Autodesk Inventor part; units mm, degrees
ref_plane "YZ Plane" through (0, 0, 0) normal (1, 0, 0) x (0, 1, 0)
ref_plane "XZ Plane" through (0, 0, 0) normal (0, 1, 0) x (-1, 0, 0)
ref_plane "XY Plane" through (0, 0, 0) normal (0, 0, 1) x (1, 0, 0)
sketch "Sketch1" plane through (0, 0, 0) normal (0, 0, 1) x (1, 0, 0)
  line L0 (-7.5, 7.5) -> (7.5, 7.5)
  line L1 (7.5, 7.5) -> (7.5, -7.5)
  line L2 (7.5, -7.5) -> (-7.5, -7.5)
  line L3 (-7.5, -7.5) -> (-7.5, 7.5)
  line L4 (-7.5, 7.5) -> (7.5, -7.5) construction
  line L5 (7.5, 7.5) -> (-7.5, -7.5) construction
  point P0 (0, 0)
  dimension "d0" = 15
  dimension "d1" = 15
extrude "Extrusion1" add sketch "Sketch1" along normal blind 2
sketch "Sketch2" plane through (0, 0, 2) normal (0, 0, 1) x (1, 0, 0)
  line L0 (-7.5, -7.5) -> (7.5, -7.5)
  line L1 (1.5, 7.5) -> (1.5, -7.5) construction
  line L2 (-1.5, -7.5) -> (-1.5, 7.5) construction
  line L3 (1.5, 7.5) -> (2, 7.5) construction
  line L4 (2, 7.5) -> (2, -7.5)
  line L5 (2, -7.5) -> (1.5, -7.5)
  line L6 (1.5, -7.5) -> (1.5, 7.5)
  line L7 (7.5, -7.5) -> (-7.5, -7.5)
  line L8 (-1.5, 7.5) -> (-2, 7.5)
  line L9 (-2, 7.5) -> (-2, -7.5)
  line L10 (-2, -7.5) -> (-1.5, -7.5)
  line L11 (-1.5, -7.5) -> (-1.5, 7.5)
  line L12 (7.5, 7.5) -> (-7.5, 7.5)
  line L13 (2, -7.5) -> (3, -7.5)
  line L14 (3, -7.5) -> (3, 7.5)
  line L15 (3, 7.5) -> (2, 7.5)
  line L16 (-2, 7.5) -> (-3, 7.5)
  line L17 (-3, 7.5) -> (-3, -7.5)
  line L18 (-2, -7.5) -> (-3, -7.5)
  point P0 (0, 0)
  dimension "d4" = 0.5
  dimension "d5" = 0.5
  dimension "d8" = 1
  dimension "d9" = 1
extrude "Extrusion2" add sketch "Sketch2" along normal blind 3 contours L17 L12 L9 L0 | L4 L12 L14 L0
equation "\"d5\" = d4"
equation "\"d9\" = d8"
equation "\"BendRadius\" = Thickness"
equation "\"BendReliefWidth\" = Thickness"
equation "\"BendReliefDepth\" = 0.5 * Thickness"
equation "\"CornerReliefSize\" = 4 * Thickness"
equation "\"MinimumRemnant\" = 2 * Thickness"
equation "\"TransitionRadius\" = BendRadius"
equation "\"JacobiRadiusSize\" = Thickness"
equation "\"GapSize\" = Thickness"
properties part number "weight_holder_base"
CAD build for the part. Positions are in the model's coordinates, mm. A direction names the side the tool comes from. Give positions to 0.01 mm unless a question says otherwise; leave off trailing zeros. Order: outer loops, then holes, each group sorted by start corner. A loop starts at its lowest first (then second) coordinate and runs counter-clockwise, first axis right, second up.
(1) Flat gauge pins, fed straight in: pin 1 (2.5 mm diameter, centred on y = 3.5, z = 4, fed in from -X); pin 2 (2 mm diameter, centred on x = -5.5, y = 2.5, fed in from +Z); pin 3 (1.5 mm diameter, centred on y = 0.5, z = 3, fed in from +X). Where does each tip first touch, or does it go through?
(2) Saw through at A-A, the plane z = 4.7. Give the cut face in (x, y), then the cut area to 3 significant figures.
(3) Saw through at C-C, the plane x = -0.25. Give the cut face in (y, z), then the cut area to 3 significant figures.
(4) Saw through at B-B, the plane y = 3.25. Give the cut face in (x, z), then the cut area to 3 significant figures.
(5) Tool access for faces 4 (the flat face through (5, 0, 2)), 5 (the flat face through (-5, 0, 2)), 6 (the flat face through (0, 0, 2)): list every direction of +Z, -Z, +X, -X, +Y, -Y with a clear straight run to the whole face (end or side of a thin tool).
(6) Mould opens along X. For faces 1 (the flat face through (7.5, 0, 1)), 2 (the flat face through (-3, 0, 3)), 3 (the flat face through (2, 0, 3)) say: released by +X, released by -X, zero draft, split by the parting line, or undercut.
(7) Drill centre lines: L1, parallel to X at y = -0.75, z = 2.45; L2, parallel to Z at x = -1, y = 3.75. Where is each one in solid material? Low to high.
Results found:
1. pin 1: stops at x = -3
1. pin 2: stops at z = 2
1. pin 3: stops at x = 3
2. outline: (-3, -7.5) - (-2, -7.5) - (-2, 7.5) - (-3, 7.5) - close; (2, -7.5) - (3, -7.5) - (3, 7.5) - (2, 7.5) - close
2. area: 30.0 mm2
3. outline: (-7.5, 0) - (7.5, 0) - (7.5, 2) - (-7.5, 2) - close
3. area: 30.0 mm2
4. outline: (-7.5, 0) - (7.5, 0) - (7.5, 2) - (3, 2) - (3, 5) - (2, 5) - (2, 2) - (-2, 2) - (-2, 5) - (-3, 5) - (-3, 2) - (-7.5, 2) - close
4. area: 36.0 mm2
5. face 4: +Z, +X, +Y, -Y
5. face 5: +Z, -X, +Y, -Y
5. face 6: +Z, +Y, -Y
6. face 1: released by +X
6. face 2: released by -X
6. face 3: undercut
7. L1: x = -3 to -2, 2 to 3
7. L2: z = 0 to 2
